Check sheet for the modelled part. Datum: model origin and axes. Units: mm. A direction names the side the tool comes from. Give positions to 0.01 mm unless a question says otherwise; leave off trailing zeros. Order: outer loops, then holes, each group sorted by start corner. A loop starts at its lowest first (then second) coordinate and runs counter-clockwise, first axis right, second up.
from build123d import *

# Parameters (mm, degrees)
SKETCH1_R           = 4.7625
SKETCH1_R_2         = 2.54
SKETCH1_R_3         = 1.5875
BOSS_EXTRUDE1_DEPTH = 12.7
SKETCH2_R           = 2.54
CUT_EXTRUDE1_DEPTH  = 9.525
SKETCH3_R           = 3.175
BOSS_EXTRUDE2_DEPTH = 38.1
SKETCH4_W           = 1.27
SKETCH4_H           = 0.762
BOSS_EXTRUDE3_DEPTH = 12.7
CUT_EXTRUDE2_START  = -15.621
CUT_EXTRUDE2_DEPTH  = 15.621


with BuildPart() as part:
    # Sketch1 → Boss-Extrude1 (new body)
    # profile 1 of 3: a face of its own
    with BuildSketch(Plane(origin=(0, 0, 0), x_dir=(0, 0, -1), z_dir=(1, 0, 0))):
        Circle(SKETCH1_R)
        Circle(SKETCH1_R_2, mode=Mode.SUBTRACT)
    # profile 2 of 3: a face of its own
    with BuildSketch(Plane(origin=(0, 0, 0), x_dir=(0, 0, -1), z_dir=(1, 0, 0))):
        Circle(SKETCH1_R_2)
        Circle(SKETCH1_R_3, mode=Mode.SUBTRACT)
    # profile 3 of 3: a face of its own
    with BuildSketch(Plane(origin=(0, 0, 0), x_dir=(0, 0, -1), z_dir=(1, 0, 0))):
        Circle(SKETCH1_R_3)
    extrude(amount=BOSS_EXTRUDE1_DEPTH)

    # Sketch2 → Cut-Extrude1 (cut)
    with BuildSketch(Plane.ZY):
        Circle(SKETCH2_R)
    extrude(amount=-CUT_EXTRUDE1_DEPTH, mode=Mode.SUBTRACT)

    # Sketch3 → Boss-Extrude2 (add)
    with BuildSketch(Plane(origin=(12.7, 0, 0), x_dir=(0, 0, -1), z_dir=(1, 0, 0))):
        with Locations(Location((0, 0, 0), (0, 0, 180))):
            Circle(SKETCH3_R)
    extrude(amount=BOSS_EXTRUDE2_DEPTH)

    # Sketch4 → Boss-Extrude3 (add)
    with BuildSketch(Plane(origin=(12.7, 0, 0), x_dir=(0, 0, -1), z_dir=(1, 0, 0))):
        with Locations((0, 4.7625)):
            Rectangle(SKETCH4_W, SKETCH4_H)
    extrude(amount=-BOSS_EXTRUDE3_DEPTH)

    # Sketch5 → Cut-Extrude2 (cut)
    with BuildSketch(Plane(origin=(50.8, 0, 0), x_dir=(0, 0, -1), z_dir=(1, 0, 0)).offset(CUT_EXTRUDE2_START)):
        with BuildLine():
            Line((-2.54, 1.905), (2.54, 1.905))
            ThreePointArc((2.54, 1.905), (0, 3.175), (-2.54, 1.905))
        make_face()
    extrude(amount=CUT_EXTRUDE2_DEPTH, mode=Mode.SUBTRACT)


solid = part.part
1) Set-up check for faces 4 (the face through (9.525, 0, 0)), 5 (the face through (12.7, -0.84, 3.24)), 6 (the face through (35.179, 2.4, 0)): record each of +Z, -Z, +X, -X, +Y, -Y from which the full face is reachable in a straight line by a thin tool's end or side.
Recorded:
face 4: -X
face 5: +X
face 6: +Z, -Z, +X, +Y
2) Section check C-C, the plane x = 25.5. Record the cut outline in (y, z) (3 decimals), then the cut area to 3 significant figures.
Recorded:
outline: circle Ø6.35 at (0, 0)
area: 31.7 mm2
3) Section check D-D, the plane z = 2. Record the cut outline in (x, y) (3 decimals).
Recorded:
outline: (0, -4.322) - (12.7, -4.322) - (12.7, -2.466) - (50.8, -2.466) - (50.8, 1.905) - (35.179, 1.905) - (35.179, 2.466) - (12.7, 2.466) - (12.7, 4.322) - (0, 4.322) - (0, 1.566) - (9.525, 1.566) - (9.525, -1.566) - (0, -1.566) - close
4) Section check A-A, the plane z = 0. Record the cut outline in (x, y) (1 decimal).
Recorded:
outline: (0, -4.8) - (12.7, -4.8) - (12.7, -3.2) - (50.8, -3.2) - (50.8, 1.9) - (35.2, 1.9) - (35.2, 3.2) - (12.7, 3.2) - (12.7, 5.1) - (0, 5.1) - (0, 2.5) - (9.5, 2.5) - (9.5, -2.5) - (0, -2.5) - close
5) Depth check by flat-ended pin: pin 1 Ø4 at (y, z) = (-0.5, 0.5) entering from -X; pin 2 Ø1.5 at (x, z) = (34, 1.5) entering from -Y; pin 3 Ø4.5 at (y, z) = (0, 0) entering from -X (3 decimals); pin 4 Ø4 at (x, z) = (41, -0.5) entering from +Y (3 decimals). Enter the tip coordinate at first touch or a pass-through.
Recorded:
pin 1: stops at x = 0
pin 2: stops at y = -3.09
pin 3: stops at x = 9.525
pin 4: stops at y = 1.905
6) Material ranges on L1, parallel to Y at x = 2.5, z = 0; L2, parallel to X at y = 2.75, z = -2.5; L3, parallel to Z at x = 7.5, y = -2, recorded low to high.
Recorded:
L1: y = -4.76 to -2.54, 2.54 to 5.14
L2: x = 0 to 12.7
L3: z = -4.32 to -1.57, 1.57 to 4.32
7) Draft check along Y on faces 1 (the face through (0, -2, -2)), 2 (the face through (6.26, -4.76, 0.2)), 3 (the face through (4.7, 2.52, -0.33)). Enter one of: +Y half, -Y half, draft (parallel to the pull), parting line (faces both ways), or undercut.
Recorded:
face 1: draft
face 2: parting line
face 3: undercut
8) Section check B-B, the plane y = 0. Record the cut outline in (x, z) (1 decimal).
Recorded:
outline: (0, -4.8) - (12.7, -4.8) - (12.7, -3.2) - (50.8, -3.2) - (50.8, 3.2) - (12.7, 3.2) - (12.7, 4.8) - (0, 4.8) - (0, 2.5) - (9.5, 2.5) - (9.5, -2.5) - (0, -2.5) - close
